from build123d import *

# Parameters (mm, degrees)
BOSS_EXTRUDE2_DEPTH = 6.35


with BuildPart() as part:
    # Elevator Ball Support Rail → Boss-Extrude2 (new body)
    with BuildSketch(Plane(origin=(0, 0, 0), x_dir=(0, 0, -1), z_dir=(1, 0, 0))):
        with BuildLine():
            ThreePointArc((0, 146.05), (24.401519846, 204.960480154), (83.312, 229.362))
            Line((83.312, 229.362), (83.312, 254.762))
            ThreePointArc((83.312, 254.762), (6.441007604, 222.920992396), (-25.4, 146.05))
            Line((-25.4, 146.05), (-25.4, 36.576))
            Line((-25.4, 36.576), (-31.75, 36.576))
            Line((-31.75, 36.576), (-31.75, 30.226))
            Line((-31.75, 30.226), (-25.4, 30.226))
            Line((-25.4, 30.226), (-25.4, 23.876))
            Line((-25.4, 23.876), (-19.865000021, 23.876))
            Line((-19.865000021, 23.876), (-19.865000021, 25.916999982))
            Line((-19.865000021, 25.916999982), (-16.964999979, 25.916999982))
            Line((-16.964999979, 25.916999982), (-16.964999979, 23.876))
            Line((-16.964999979, 23.876), (-11.43, 23.876))
            Line((-11.43, 23.876), (-11.43, 19.558))
            Line((-11.43, 19.558), (-16.964999979, 19.558))
            Line((-16.964999979, 19.558), (-16.964999979, 17.517000018))
            Line((-16.964999979, 17.517000018), (-19.865000021, 17.517000018))
            Line((-19.865000021, 17.517000018), (-19.865000021, 19.558))
            Line((-19.865000021, 19.558), (-25.4, 19.558))
            Line((-25.4, 19.558), (-25.4, 13.208))
            Line((-25.4, 13.208), (-31.75, 13.208))
            Line((-31.75, 13.208), (-31.75, 6.858))
            Line((-31.75, 6.858), (-25.4, 6.858))
            Line((-25.4, 6.858), (-25.4, -90.424))
            Line((-25.4, -90.424), (-31.75, -90.424))
            Line((-31.75, -90.424), (-31.75, -96.774))
            Line((-31.75, -96.774), (-25.4, -96.774))
            Line((-25.4, -96.774), (-25.4, -103.124))
            Line((-25.4, -103.124), (-19.865000021, -103.124))
            Line((-19.865000021, -103.124), (-19.865000021, -101.083000018))
            Line((-19.865000021, -101.083000018), (-16.964999979, -101.083000018))
            Line((-16.964999979, -101.083000018), (-16.964999979, -103.124))
            Line((-16.964999979, -103.124), (-11.43, -103.124))
            Line((-11.43, -103.124), (-11.43, -107.442))
            Line((-11.43, -107.442), (-16.964999979, -107.442))
            Line((-16.964999979, -107.442), (-16.964999979, -109.482999982))
            Line((-16.964999979, -109.482999982), (-19.865000021, -109.482999982))
            Line((-19.865000021, -109.482999982), (-19.865000021, -107.442))
            Line((-19.865000021, -107.442), (-25.4, -107.442))
            Line((-25.4, -107.442), (-25.4, -113.792))
            Line((-25.4, -113.792), (-31.75, -113.792))
            Line((-31.75, -113.792), (-31.75, -120.142))
            Line((-31.75, -120.142), (-25.4, -120.142))
            Line((-25.4, -120.142), (-25.4, -146.05))
            ThreePointArc((-25.4, -146.05), (-37.346353976, -168.922761976), (-61.468, -178.08926659))
            Line((-61.468, -178.08926659), (-61.468, -196.342))
            Line((-61.468, -196.342), (-61.468, -202.692))
            Line((-61.468, -202.692), (-55.118, -202.692))
            Line((-55.118, -202.692), (-55.118, -196.342))
            Line((-55.118, -196.342), (-48.768, -196.342))
            Line((-48.768, -196.342), (-48.768, -190.807000021))
            Line((-48.768, -190.807000021), (-50.808999982, -190.807000021))
            Line((-50.808999982, -190.807000021), (-50.808999982, -187.906999979))
            Line((-50.808999982, -187.906999979), (-48.768, -187.906999979))
            Line((-48.768, -187.906999979), (-48.768, -182.372))
            Line((-48.768, -182.372), (-44.45, -182.372))
            Line((-44.45, -182.372), (-44.45, -187.906999979))
            Line((-44.45, -187.906999979), (-42.409000018, -187.906999979))
            Line((-42.409000018, -187.906999979), (-42.409000018, -190.807000021))
            Line((-42.409000018, -190.807000021), (-44.45, -190.807000021))
            Line((-44.45, -190.807000021), (-44.45, -196.342))
            Line((-44.45, -196.342), (-38.1, -196.342))
            Line((-38.1, -196.342), (-38.1, -202.692))
            Line((-38.1, -202.692), (-31.75, -202.692))
            Line((-31.75, -202.692), (-31.75, -196.342))
            Line((-31.75, -196.342), (-23.236080339, -196.342))
            ThreePointArc((-23.236080339, -196.342), (-13.043034257, -213.854764297), (0, -229.362))
            Line((0, -229.362), (83.312, -229.362))
            ThreePointArc((83.312, -229.362), (24.401519846, -204.960480154), (0, -146.05))
            Line((0, -146.05), (0, 146.05))
        make_face()
    extrude(amount=BOSS_EXTRUDE2_DEPTH)


solid = part.part
Verification items for the finished model (mm, model axes). A direction names the side the tool comes from. Give positions to 0.01 mm unless a question says otherwise; leave off trailing zeros. Loops run counter-clockwise (first coordinate to the right, second up) from the corner with the lowest first, then second, coordinate; pieces in that order, holes last.
1) Draft check along Y on faces 4 (the cylindrical face through (3.13, 223.76, -7.29)), 5 (the cylindrical face through (3.1, -168.7, 37.1)), 6 (the flat face through (6.35, -4, 6)). Enter one of: pulls with the +Y half, pulls with the -Y half, needs draft (parallel to the pull), parting line crosses it, or undercut.
2) Depth check by flat-ended pin: pin 1 Ø1.9 at (x, z) = (4.5, 28.5) entering from +Y; pin 2 Ø1 at (x, z) = (3, -51) entering from +Y; pin 3 Ø1.6 at (x, y) = (4.5, 18.5) entering from +Z; pin 4 Ø12 at (y, z) = (-40, 33) entering from -X. Enter the tip coordinate at first touch or a pass-through.
3) Set-up check for faces 1 (the cylindrical face through (3.13, -213.62, 13.21)), 2 (the flat face through (0, -4, 6)), 3 (the cylindrical face through (3.13, 204.31, -23.76)): record each of +Z, -Z, +X, -X, +Y, -Y from which the full face is reachable in a straight line by a thin tool's end or side.
4) Sectioned sample at A-A, the plane z = -56.5. Enter the section's corners in (x, y).
5) Sectioned sample at B-B, the plane y = -77.5. Enter the section's corners in (x, z).
6) Thickness scan on line 1 along Y through (x, z) = (5.75, 17); line 2 along Z through (x, y) = (0.5, -74); line 3 along Y through (x, z) = (5.5, -35). Record the ranges inside material, lowest first.
7) Sectioned sample at C-C, the plane y = 162. Enter the section's corners in (x, z), then the cut area to 3 significant figures.
Answers:
1. face 4: pulls with the +Y half
1. face 5: undercut
1. face 6: needs draft
2. pin 1: stops at y = 36.58
2. pin 2: stops at y = 250
2. pin 3: stops at z = 25.4
2. pin 4: passes through
3. face 1: +X, -X, -Y
3. face 2: +Z, -Z, -X, +Y, -Y
3. face 3: -Z, +X, -X
4. outline: (0, -229.36) - (6.35, -229.36) - (6.35, -224.93) - (0, -224.93) - close; (0, 224.93) - (6.35, 224.93) - (6.35, 251.4) - (0, 251.4) - close
5. outline: (0, 0) - (6.35, 0) - (6.35, 25.4) - (0, 25.4) - close
6. line 1: y = -207.85 to -109.48, -101.08 to 17.52, 25.92 to 187.95
6. line 2: z = 0 to 25.4
6. line 3: y = -229.36 to -213.92, 213.92 to 243.44
7. outline: (0, -1.54) - (6.35, -1.54) - (6.35, 24.22) - (0, 24.22) - close
7. area: 164 mm2
